```python
from build123d import *

# Parameters (mm, degrees)
SKETCH1_W           = 40
SKETCH1_H           = 35
BOSS_EXTRUDE1_DEPTH = 1.6
SKETCH2_R           = 1.45
SKETCH2_W           = 26
SKETCH2_H           = 24
CUT_EXTRUDE1_DEPTH  = 27.623485872
SKETCH4_W           = 60
SKETCH4_H           = 7.921096837
BOSS_EXTRUDE2_DEPTH = 1.6
SKETCH3_R           = 1.7
CUT_EXTRUDE2_DEPTH  = 82.90732568
FILLET1_R           = 1


with BuildPart() as part:
    # Sketch1 → Boss-Extrude1 (new body)
    with BuildSketch(Plane(origin=(0, 0, 0), x_dir=(1, 0, 0), z_dir=(0, 1, 0))):
        Rectangle(SKETCH1_W, SKETCH1_H)
    extrude(amount=BOSS_EXTRUDE1_DEPTH)

    # Sketch2 → Cut-Extrude1 (cut, through all)
    with BuildSketch(Plane(origin=(0, 1.6, 0), x_dir=(1, 0, 0), z_dir=(0, 1, 0))):
        with Locations(Location((-16.5, 3.5, 0), (0, 0, 270))):
            Circle(SKETCH2_R)
        with Locations(Location((-16.5, -14, 0), (0, 0, 270))):
            Circle(SKETCH2_R)
        with Locations(Location((16.5, 3.5, 0), (0, 0, 270))):
            Circle(SKETCH2_R)
        with Locations(Location((16.5, -14, 0), (0, 0, 270))):
            Circle(SKETCH2_R)
        with Locations((0, -5.5)):
            Rectangle(SKETCH2_W, SKETCH2_H)
    extrude(amount=-CUT_EXTRUDE1_DEPTH, mode=Mode.SUBTRACT)

    # Sketch4 → Boss-Extrude2 (add)
    with BuildSketch(Plane.XZ):
        with Locations((-50, -13.539451581)):
            Rectangle(SKETCH4_W, SKETCH4_H)
    extrude(amount=-BOSS_EXTRUDE2_DEPTH)

    # Sketch3 → Cut-Extrude2 (cut, through all)
    with BuildSketch(Plane(origin=(0, 1.6, 0), x_dir=(1, 0, 0), z_dir=(0, 1, 0))):
        with Locations(Location((16, 13.5, 0), (0, 0, 270))):
            Circle(SKETCH3_R)
        with Locations(Location((-76, 13.5, 0), (0, 0, 270))):
            Circle(SKETCH3_R)
    extrude(amount=-CUT_EXTRUDE2_DEPTH, mode=Mode.SUBTRACT)

    # Fillet1
    fillet1_edges = [part.edges().sort_by_distance(p)[0] for p in [
        (-13, 0.8, 17.5),
        (13, 0.8, 17.5),
        (-80, 0.8, -17.5),
        (-80, 0.8, -9.578903163),
        (20, 0.8, 17.5),
        (-20, 0.8, 17.5),
        (20, 0.8, -17.5),
    ]]
    fillet(fillet1_edges, radius=FILLET1_R)


solid = part.part
```
Work out the finished part from the listing and answer in its coordinate system (mm). A direction names the side the tool comes from. Round coordinates to 2 decimals unless told otherwise and drop trailing zeros. Loops run counter-clockwise (first coordinate to the right, second up) from the corner with the lowest first, then second, coordinate; pieces in that order, holes last. Notation, with made-up numbers: M -33,43 L -14,43 A19 cw -14,51 Z; hole C -17.5,-34 d11. An arc over 180 degrees is marked long. One line per question, with ' | ' between items.
Q1. Find section A-A, the plane z = -13.5. Give the vertices of the cut face in (x, y).
Conclusion:
outline: M -80,0 L -77.7,0 L -77.7,1.6 L -80,1.6 Z; M -74.3,0 L 14.3,0 L 14.3,1.6 L -74.3,1.6 Z; M 17.7,0 L 20,0 L 20,1.6 L 17.7,1.6 Z
Q2. A tool of negligible diameter and unlimited length cuts with its end or side. For faces 5 (the flat face through (-20, 1, 4)), 6 (the flat face through (-31, 1, -17.5)), 7 (the flat face through (13, 1, 5)), from which of +Z, -Z, +X, -X, +Y, -Y can it reach the whole face along a straight path? Write none if from no direction.
Conclusion:
face 5: +Z, -X, +Y, -Y | face 6: -Z, +X, -X, +Y, -Y | face 7: +Z, +Y, -Y
Q3. Consider line 1 along X through (y, z) = (0.7, 14); line 2 along X through (y, z) = (1, -13.5); line 3 along X through (y, z) = (0.15, 7). Determine where each line is inside the solid, lowest interval first. Write a range as from..to.
Conclusion:
line 1: x = -20..-17.95, -15.05..-13, 13..15.05, 17.95..20 | line 2: x = -80..-77.7, -74.3..14.3, 17.7..20 | line 3: x = -20..-13, 13..20
Q4. Find section D-D, the plane x = -76. Give the vertices of the cut face in (y, z), then the cut area to 3 significant figures.
Conclusion:
outline: M 0,-17.5 L 1.6,-17.5 L 1.6,-15.2 L 0,-15.2 Z; M 0,-11.8 L 1.6,-11.8 L 1.6,-9.58 L 0,-9.58 Z | area: 7.23 mm2
Q5. Find section C-C, the plane z = 0. Give the vertices of the cut face in (x, y).
Conclusion:
outline: M -20,0 L -13,0 L -13,1.6 L -20,1.6 Z; M 13,0 L 20,0 L 20,1.6 L 13,1.6 Z
Q6. The mould has two halves that part along X. Classify faces 1 (the cylindrical face through (15.62, 0.81, -4.65)), 2 (the flat face through (0, 1, -6.5)), 3 (the flat face through (-80, 1, -14)), 4 (the flat face through (-17, 1, 17.5)): +X half, -X half, draft (parallel to the pull), parting line (faces both ways), or undercut.
Conclusion:
face 1: undercut | face 2: undercut | face 3: -X half | face 4: draft
Q7. Find section B-B, the plane y = 1.25. Give the vertices of the cut face in (x, z), then the cut area to 3 significant figures.
Conclusion:
outline: M -80,-16.5 A1 ccw -79,-17.5 L 19,-17.5 A1 ccw 20,-16.5 L 20,16.5 A1 ccw 19,17.5 L 14,17.5 A1 ccw 13,16.5 L 13,-6.5 L -13,-6.5 L -13,16.5 A1 ccw -14,17.5 L -19,17.5 A1 ccw -20,16.5 L -20,-9.58 L -79,-9.58 A1 ccw -80,-10.58 Z; hole C -76,-13.5 d3.4; hole C -16.5,-3.5 d2.9; hole C -16.5,14 d2.9; hole C 16,-13.5 d3.4; hole C 16.5,-3.5 d2.9; hole C 16.5,14 d2.9 | area: 1,210 mm2
Q8. Each of these flat-tipped pins is pushed along its axis until it touches: pin 1 Ø2.5 at (x, z) = (16, -13.5) entering from -Y; pin 2 Ø0.5 at (y, z) = (0.5, 10) entering from -X; pin 3 Ø0.8 at (x, y) = (1, 1) entering from +Z. Where does it stop, or does it pass through?
Conclusion:
pin 1: passes through | pin 2: stops at x = -20 | pin 3: stops at z = -6.5
